The listing builds one solid part. Answer for the finished solid, in the listing's coordinates (mm). Give positions to 0.01 mm unless a question says otherwise; leave off trailing zeros. Loops run counter-clockwise (first coordinate to the right, second up) from the corner with the lowest first, then second, coordinate; pieces in that order, holes last. Notation, with made-up numbers: M 10.25,67 L 46.25,67 A8 cw 46.25,76 Z; hole C -16.5,58 d6. An arc over 180 degrees is marked long. Return JSON: item names as keys, results as strings.
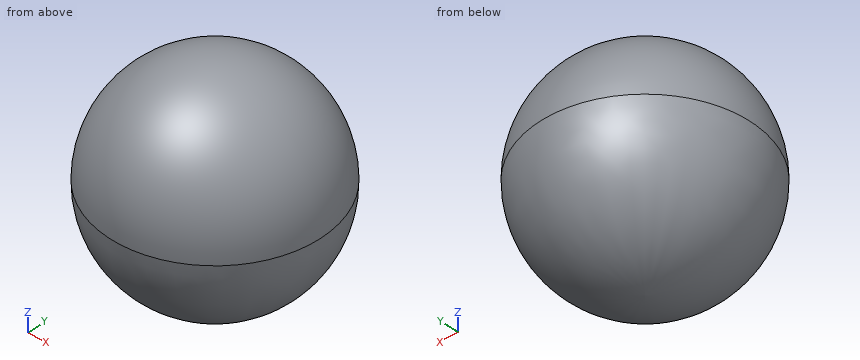
from build123d import *

# Parameters (mm, degrees)
F0_R     = 7.5
F1_DEPTH = 7.5
F2_R     = 7.5
F3_R     = 7.49999


# Not quite as in the source:
# - a fillet or chamfer is up to 0.001 mm smaller than in the source, because OpenCascade refuses the exact size


with BuildPart() as f1:
    # F0 (on Top) → F1 (new body, symmetric)
    with BuildSketch(Plane.XY):
        Circle(F0_R)
    extrude(amount=F1_DEPTH, both=True)

    # F2
    f2_edges = [f1.edges().sort_by_distance(p)[0] for p in [
        (-7.5, 0, 7.5),
    ]]
    fillet(f2_edges, radius=F2_R)

    # F3 (radius 7.5 in the source; OpenCascade refuses exactly that, so slightly less here)
    f3_edges = [f1.edges().sort_by_distance(p)[0] for p in [
        (-7.5, 0, -7.5),
    ]]
    fillet(f3_edges, radius=F3_R)


solid = f1.part
(1) Given pin 1 (4 mm diameter, centred on x = 5, z = -3, fed in from +Y); pin 2 (1.5 mm diameter, centred on x = 3, y = 4.5, fed in from -Z); pin 3 (2 mm diameter, centred on x = 3, y = -3.5, fed in from +Z), each flat-ended and moving along its own axis, determine where each tip first touches the part or whether it passes through.
Values follow:
{"pin 1": "y = 6.45", "pin 2": "z = -5.88", "pin 3": "z = 6.57"}
(2) The part is cut by section A-A (z = 2.25). Determine the outline of the cut face in (x, y), and give its area (3 significant figures).
Values follow:
{"outline": "C 0,0 d14.31", "area": "161 mm²"}
(3) Straight lines are drawn through the part: line 1 along Z through (x, y) = (6.5, -1.5); line 2 along Z through (x, y) = (-6.5, -0.25). For each, find the intervals that lie inside material, in ascending order.
Values follow:
{"line 1": "-3.43 to 3.43", "line 2": "-3.73 to 3.73"}
(4) The part is cut by section B-B (z = 5.5). Determine the outline of the cut face in (x, y), and give its area (3 significant figures).
Values follow:
{"outline": "C 0,0 d10.2", "area": "81.7 mm²"}
